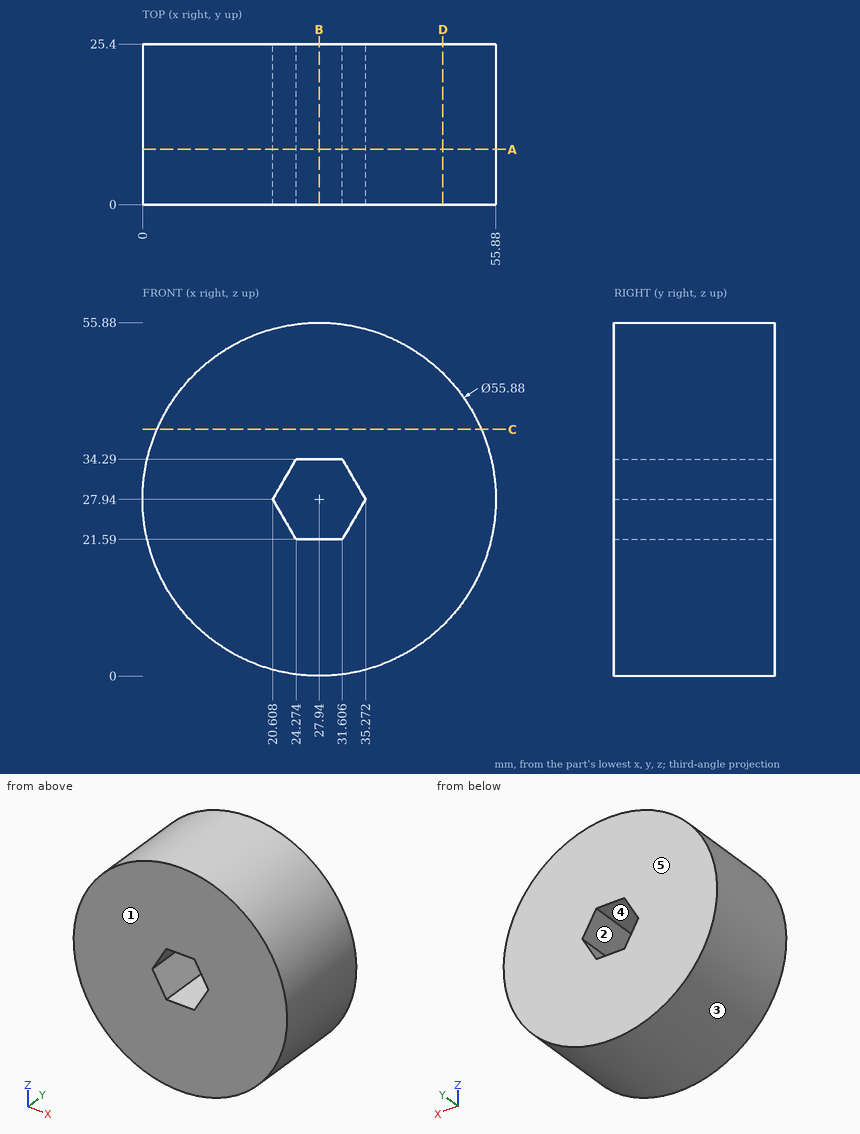
Geometry check sheet. Reference: drawing and pictorial views, mm from the part's lowest x, y, z. A direction names the side the tool comes from. Round coordinates to 2 decimals unless told otherwise and drop trailing zeros. Write each loop counter-clockwise with the first axis right and the second up, starting at its lowest first coordinate (ties: lowest second). Pieces come first, ordered by that corner, then holes.
1. Section check D-D on x = 47.5. Enter the section's corners in (y, z).
2. Scan lines: L1, parallel to Z at x = 27, y = 19; L2, parallel to Z at x = 29.5, y = 3.75; L3, parallel to X at y = 11, z = 28. Record each from-to range of solid material in increasing order.
3. Section check C-C on z = 39. Enter the section's corners in (x, y), plus the area to 3 significant figures.
4. Access from +Z, -Z, +X, -X, +Y, -Y to the whole of each face (thin tool, end or side, straight path). Record for the marked faces 4 and 5.
5. Gauge pin test, flat ends, axial feed: P1, Ø4, axis at y = 21, z = 17.5, coming from the -X side (1 decimal); P2, Ø8, axis at x = 21, y = 5.5, coming from the -Z side (1 decimal); P3, Ø3, axis at y = 15, z = 44, coming from the -X side. Record the tip position at first contact, or that the pin passes through.
6. Draft check along X on the marked faces 1, 2 and 3. Enter one of: +X half, -X half, draft (parallel to the pull), parting line (faces both ways), or undercut.
7. Section check B-B on x = 27.94. Enter the section's corners in (y, z).
8. Section check A-A on y = 8.75. Enter the section's corners in (x, z).
Answer:
1. outline: (0, 7.99) - (25.4, 7.99) - (25.4, 47.89) - (0, 47.89) - close
2. L1: z = 0.02 to 21.59, 34.29 to 55.86
2. L2: z = 0.04 to 21.59, 34.29 to 55.84
2. L3: x = 0 to 20.64, 35.24 to 55.88
3. outline: (2.28, 0) - (53.6, 0) - (53.6, 25.4) - (2.28, 25.4) - close
3. area: 1,300 mm2
4. face 4: +Y, -Y
4. face 5: +Z, -Z, +X, -X, +Y
5. P1: stops at x = 1.3
5. P2: stops at z = 0.2
5. P3: stops at x = 4.09
6. face 1: draft
6. face 2: undercut
6. face 3: parting line
7. outline: (0, 0) - (25.4, 0) - (25.4, 21.59) - (0, 21.59) - close; (0, 34.29) - (25.4, 34.29) - (25.4, 55.88) - (0, 55.88) - close
8. outline: circle Ø55.88 at (27.94, 27.94); hole (20.61, 27.94) - (24.27, 21.59) - (31.61, 21.59) - (35.27, 27.94) - (31.61, 34.29) - (24.27, 34.29) - close
